CAD build for the part. Positions are in the model's coordinates, mm. A direction names the side the tool comes from. Round coordinates to 2 decimals unless told otherwise and drop trailing zeros. Order: outer loops, then holes, each group sorted by start corner. A loop starts at its lowest first (then second) coordinate and runs counter-clockwise, first axis right, second up. Notation, with made-up numbers: (25.25, -20) - (49.25, -20) arc R19 ccw to (49.25, 15) - close; hole circle Ø4 at (-30, 7). An arc over 180 degrees is marked (long way). Write item = value, one per line.
from build123d import *

# Parameters (mm, degrees)
PCB_DEPTH                = 1.5
ESQUISSE3_R              = 1
ESQUISSE3_R_2            = 0.75
TROUS_DEPTH              = 42.788156217
M3_CLEARANCE_HOLE2_D     = 3.2
M3_CLEARANCE_HOLE2_DEPTH = 5
M3_CLEARANCE_HOLE2_TIP   = 0.96137699


with BuildPart() as part:
    # Esquisse2 → PCB (new body)
    with BuildSketch(Plane.XY):
        with BuildLine():
            Line((-10, 0), (-2, 0))
            ThreePointArc((-2, 0), (0, -2), (2, 0))
            Line((2, 0), (10, 0))
            Line((10, 0), (10, 7.5))
            ThreePointArc((10, 7.5), (7.5, 10), (10, 12.5))
            Line((10, 12.5), (10, 28))
            ThreePointArc((10, 28), (12, 30), (10, 32))
            Line((10, 32), (10, 40))
            Line((10, 40), (2.5, 40))
            ThreePointArc((2.5, 40), (0, 37.5), (-2.5, 40))
            Line((-2.5, 40), (-10, 40))
            Line((-10, 40), (-10, 32))
            ThreePointArc((-10, 32), (-12, 30), (-10, 28))
            Line((-10, 28), (-10, 12.5))
            ThreePointArc((-10, 12.5), (-7.5, 10), (-10, 7.5))
            Line((-10, 7.5), (-10, 0))
        make_face()
    extrude(amount=PCB_DEPTH)

    # Esquisse3 → Trous (cut, through all)
    with BuildSketch(Plane.XY.offset(1.5)):
        with Locations((-10, 30)):
            Circle(ESQUISSE3_R)
        with Locations((6.37737312, 1.435143304)):
            Circle(ESQUISSE3_R_2)
        with Locations(Location((10, 30, 0), (0, 0, 180))):
            Circle(ESQUISSE3_R)
        Circle(ESQUISSE3_R)
        with Locations((3.809466202, 1.435143304)):
            Circle(ESQUISSE3_R_2)
        with Locations((-4.012518268, 1.435143304)):
            Circle(ESQUISSE3_R_2)
        with Locations((-6.688956118, 1.435143304)):
            Circle(ESQUISSE3_R_2)
    extrude(amount=-TROUS_DEPTH, mode=Mode.SUBTRACT)

    # M3 Clearance Hole2
    with Locations(Plane(origin=(0, 0, 0), x_dir=(-1, 0, 0), z_dir=(0, 0, -1))):
        with Locations((0, 12.3952)):
            Hole(M3_CLEARANCE_HOLE2_D / 2, depth=M3_CLEARANCE_HOLE2_DEPTH)
            with Locations((0, 0, -(M3_CLEARANCE_HOLE2_DEPTH + M3_CLEARANCE_HOLE2_TIP / 2))):  # 118° drill point
                Cone(0, M3_CLEARANCE_HOLE2_D / 2, M3_CLEARANCE_HOLE2_TIP, mode=Mode.SUBTRACT)


solid = part.part
(1) Tool access for faces 5 (the cylindrical face through (-12, 30, 1)), 6 (the flat face through (-10, 20, 1)), 7 (the flat face through (10, 4, 1)): list every direction of +Z, -Z, +X, -X, +Y, -Y with a clear straight run to the whole face (end or side of a thin tool).
Solved:
face_5 = +Z, -Z, -X
face_6 = +Z, -Z, -X, -Y
face_7 = +Z, -Z, +X, -Y
(2) Drop flat-ended pins along their axis: pin 1 (0.8 mm diameter, centred on x = 5.5, z = 1, fed in from -Y); pin 2 (0.8 mm diameter, centred on y = 34, z = 0.5, fed in from +X). Give the stop position or say it passes through.
Solved:
pin_1 = 0
pin_2 = 10
(3) Pull direction X, two halves, no side cores. Call faces 1 (the cylindrical face through (4.525, 1.66, 0.76)), 2 (the flat face through (-10, 4, 1)), 3 (the flat face through (6, 40, 1)), 4 (the cylindrical face through (-4.11, 2.18, 0.76)): released by +X, released by -X, zero draft, split by the parting line, or undercut.
Solved:
face_1 = undercut
face_2 = released by -X
face_3 = zero draft
face_4 = undercut
(4) Band-saw the part on A-A on y = 30. List the corners of the cut face in (x, z).
Solved:
outline = (-12, 0) - (-11, 0) - (-11, 1.5) - (-12, 1.5) - close; (-9, 0) - (9, 0) - (9, 1.5) - (-9, 1.5) - close; (11, 0) - (12, 0) - (12, 1.5) - (11, 1.5) - close
(5) Band-saw the part on B-B on x = 0. List the corners of the cut face in (y, z).
Solved:
outline = (-2, 0) - (-1, 0) - (-1, 1.5) - (-2, 1.5) - close; (1, 0) - (10.8, 0) - (10.8, 1.5) - (1, 1.5) - close; (14, 0) - (37.5, 0) - (37.5, 1.5) - (14, 1.5) - close
(6) Band-saw the part on C-C on x = -7. List the corners of the cut face in (y, z).
Solved:
outline = (0, 0) - (0.75, 0) - (0.75, 1.5) - (0, 1.5) - close; (2.12, 0) - (40, 0) - (40, 1.5) - (2.12, 1.5) - close
(7) Band-saw the part on D-D on z = 0.4. Count the separate pieces of the cut face and the enclosed holes in it, plus the area to 3 significant figures.
Solved:
separate_pieces = 1
enclosed_holes = 8
area = 765 mm²
(8) Probe line 1 along Y through (x, z) = (0, 1.2); line 2 along Y through (x, z) = (-0.5, 1.05); line 3 along Y through (x, z) = (7.25, 0.85). List the from-to ranges inside material, lowest first.
Solved:
line_1 = -2 to -1, 1 to 10.8, 14 to 37.5
line_2 = -1.94 to -0.87, 0.87 to 10.88, 13.92 to 37.55
line_3 = 0 to 40
